from build123d import *

# Parameters (mm, degrees)
SKETCH_1_R                      = 7.5
SKETCH_1_R_2                    = 2.5
EXTRUDE_1_DEPTH                 = 20
SKETCH_2_R                      = 40.75
SKETCH_2_R_2                    = 2.5
EXTRUDE_2_DEPTH                 = 5
EXTRUDE_T_DEPTH                 = 10
EXTRUDE_T_DEPTH_BACK            = 15
SKETCH_3_R                      = 40.75
SKETCH_3_R_2                    = 36.75
SKETCH_4_W                      = 20
SKETCH_4_H                      = 17.5
EXTRUDE_4_DEPTH                 = 70
SKETCH_6_W                      = 8
SKETCH_6_H                      = 17.5
CUT_EXTRUDE_5_DEPTH             = 40
CUT_EXTRUDE_6_REACH             = 101.303
SKETCH_7_R                      = 2.5
CUT_EXTRUDE_7_REACH             = 96.584
SKETCH_8_W                      = 71.008802272
SKETCH_8_H                      = 20.75
CUT_EXTRUDE_7_DIRECTION_2_REACH = 96.584
CUT_EXTRUDE_START               = -55
SKETCH_9_W                      = 20
SKETCH_9_H                      = 5
CUT_EXTRUDE_8_DEPTH             = 55


with BuildPart() as part:
    # Эскиз1 → Вытянуть1 (new body)
    with BuildSketch(Plane(origin=(0, 0, 0), x_dir=(1, 0, 0), z_dir=(0, 1, 0))):
        with Locations(Location((0, 0, 0), (0, 0, 270))):
            Circle(SKETCH_1_R)
        with Locations(Location((0, 0, 0), (0, 0, 270))):
            Circle(SKETCH_1_R_2, mode=Mode.SUBTRACT)
    extrude(amount=EXTRUDE_1_DEPTH)

    # Эскиз2 → Вытянуть2 (add)
    with BuildSketch(Plane(origin=(0, 0, 0), x_dir=(1, 0, 0), z_dir=(0, 1, 0))):
        with Locations(Location((0, 0, 0), (0, 0, 270))):
            Circle(SKETCH_2_R)
        with Locations(Location((0, 0, 0), (0, 0, 270))):
            Circle(SKETCH_2_R_2, mode=Mode.SUBTRACT)
    extrude(amount=EXTRUDE_2_DEPTH)

    # Эскиз3 → t (add, two sides: drawn at the far end of the back side and taken through both)
    with BuildSketch(Plane(origin=(0, 5, 0), x_dir=(1, 0, 0), z_dir=(0, 1, 0)).offset(-EXTRUDE_T_DEPTH_BACK)):
        with Locations(Location((0, 0, 0), (0, 0, 270))):
            Circle(SKETCH_3_R)
        with Locations(Location((0, 0, 0), (0, 0, 270))):
            Circle(SKETCH_3_R_2, mode=Mode.SUBTRACT)
    extrude(amount=EXTRUDE_T_DEPTH + EXTRUDE_T_DEPTH_BACK)

    # Эскиз4 → Вытянуть4 (add)
    with BuildSketch(Plane(origin=(0, 5, 0), x_dir=(1, 0, 0), z_dir=(0, 1, 0))):
        with Locations((0, 11.25)):
            Rectangle(SKETCH_4_W, SKETCH_4_H)
    extrude(amount=EXTRUDE_4_DEPTH)

    # Эскиз6 → Вытянуть5 (cut)
    with BuildSketch(Plane(origin=(0, 75, 0), x_dir=(1, 0, 0), z_dir=(0, 1, 0))):
        with Locations((0, 11.25)):
            Rectangle(SKETCH_6_W, SKETCH_6_H)
    extrude(amount=-CUT_EXTRUDE_5_DEPTH, mode=Mode.SUBTRACT)

    # Вытянуть6: up to this face of the body (flat: up to its plane)
    cut_extrude_6_end = Plane(part.part.faces().sort_by_distance((-10, 40, -11.25))[0])
    # Эскиз7 → Вытянуть6 (cut, up to the picked face)
    with BuildSketch(Plane(origin=(10, 0, 0), x_dir=(0, 0, -1), z_dir=(1, 0, 0)), mode=Mode.PRIVATE) as cut_extrude_6_sk1:
        with Locations((13.75, 45)):
            Circle(SKETCH_7_R)
    cut_extrude_6_tool1 = split(extrude(cut_extrude_6_sk1.sketch, amount=-CUT_EXTRUDE_6_REACH, mode=Mode.PRIVATE), bisect_by=cut_extrude_6_end, keep=Keep.BOTH, mode=Mode.PRIVATE)
    add(cut_extrude_6_tool1.solids().sort_by(Axis((10, 45, -13.75), (-1, 0, 0)))[0], mode=Mode.SUBTRACT)

    # Эскиз8 → Вытянуть7 (cut, up to next)
    with BuildSketch(Plane(origin=(0, 0, 0), x_dir=(1, 0, 0), z_dir=(0, 1, 0)), mode=Mode.PRIVATE) as cut_extrude_7_sk1:
        with Locations((0, 30.375)):
            Rectangle(SKETCH_8_W, SKETCH_8_H)
    cut_extrude_7_tool1 = extrude(cut_extrude_7_sk1.sketch, amount=CUT_EXTRUDE_7_REACH, mode=Mode.PRIVATE) & part.part
    add(cut_extrude_7_tool1.solids().sort_by_distance((0, 0, -30.375))[0], mode=Mode.SUBTRACT)

    # Эскиз8 → Вытянуть7 direction 2 (cut, up to next)
    with BuildSketch(Plane(origin=(0, 0, 0), x_dir=(1, 0, 0), z_dir=(0, 1, 0)), mode=Mode.PRIVATE) as cut_extrude_7_direction_2_sk1:
        with Locations((0, 30.375)):
            Rectangle(SKETCH_8_W, SKETCH_8_H)
    cut_extrude_7_direction_2_tool1 = extrude(cut_extrude_7_direction_2_sk1.sketch, amount=-CUT_EXTRUDE_7_DIRECTION_2_REACH, mode=Mode.PRIVATE) & part.part
    add(cut_extrude_7_direction_2_tool1.solids().sort_by_distance((0, 0, -30.375))[0], mode=Mode.SUBTRACT)

    # Эскиз9 → Вытянуть8 (cut)
    with BuildSketch(Plane(origin=(0, 75, 0), x_dir=(1, 0, 0), z_dir=(0, 1, 0)).offset(CUT_EXTRUDE_START)):
        with Locations((0, 5)):
            Rectangle(SKETCH_9_W, SKETCH_9_H)
    extrude(amount=CUT_EXTRUDE_8_DEPTH, mode=Mode.SUBTRACT)


solid = part.part
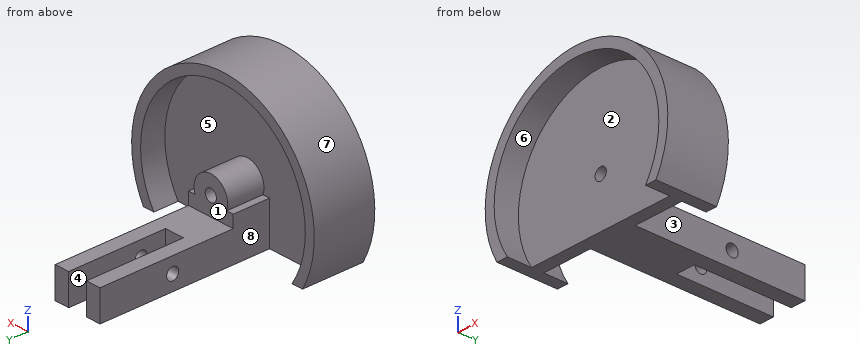
Model file for the job. Use its own axes, mm. Face numbers are marked on the shaded views. A direction names the side the tool comes from. Give positions to 0.01 mm unless a question says otherwise; leave off trailing zeros. Order: outer loops, then holes, each group sorted by start corner. A loop starts at its lowest first (then second) coordinate and runs counter-clockwise, first axis right, second up. Notation, with made-up numbers: (57.25, 88.5) - (114.25, 88.5) arc R29 cw to (114.25, 124.5) - close; hole circle Ø5 at (45.5, 77). An arc over 180 degrees is marked (long way). Return JSON: item names as keys, results as strings.
1) Cut at D-D, the plane z = -13.75. Give the cut face in (x, y), plus the area to 3 significant figures.
Geometry says:
{"outline": "(-38.36, -10) - (-34.08, -10) - (-34.08, 0) - (34.08, 0) - (34.08, -10) - (38.36, -10) - (38.36, 15) - (34.08, 15) - (34.08, 5) - (10, 5) - (10, 42.5) - (4, 42.5) - (4, 35) - (-4, 35) - (-4, 42.5) - (-10, 42.5) - (-10, 5) - (-34.08, 5) - (-34.08, 15) - (-38.36, 15) - close; (-10, 47.5) - (-4, 47.5) - (-4, 75) - (-10, 75) - close; (4, 47.5) - (10, 47.5) - (10, 75) - (4, 75) - close", "area": "1,570 mm²"}
2) Flat gauge pins, fed straight in: P1, Ø22, axis at x = 1, y = 43.5, coming from the +Z side; P2, Ø5, axis at y = 44.5, z = -11.5, coming from the +X side; P3, Ø4, axis at x = 0.5, z = -13, coming from the +Y side. Where does each tip first touch, or does it go through?
Geometry says:
{"P1": "z = -7.5", "P2": "x = 10", "P3": "y = 35"}
3) 3-axis set-ups, long thin cutter, end or side, ignore diameter. For the marked faces 1, 2, 3, 4 and 5: which of +Z, -Z, +X, -X, +Y, -Y reach the whole face in a straight line?
Geometry says:
{"face 1": "+Z, +X, -X, +Y", "face 2": "-Y", "face 3": "-Z, +Y", "face 4": "+Z, -Z, +Y", "face 5": "+Y"}
4) Cut at C-C, the plane y = 53. Give the cut face in (x, z).
Geometry says:
{"outline": "(-10, -20) - (-4, -20) - (-4, -7.5) - (-10, -7.5) - close; (4, -20) - (10, -20) - (10, -7.5) - (4, -7.5) - close"}
5) Cut at B-B, the plane z = 0. Give the cut face in (x, y).
Geometry says:
{"outline": "(-40.75, -10) - (-36.75, -10) - (-36.75, 0) - (-2.5, 0) - (-2.5, 20) - (-7.5, 20) - (-7.5, 5) - (-36.75, 5) - (-36.75, 15) - (-40.75, 15) - close; (2.5, 0) - (36.75, 0) - (36.75, -10) - (40.75, -10) - (40.75, 15) - (36.75, 15) - (36.75, 5) - (7.5, 5) - (7.5, 20) - (2.5, 20) - close"}
6) Pull direction Z, two halves, no side cores. Call the marked faces 6, 7 and 8: pulls with the +Z half, pulls with the -Z half, needs draft (parallel to the pull), parting line crosses it, or undercut.
Geometry says:
{"face 6": "undercut", "face 7": "parting line crosses it", "face 8": "needs draft"}
7) Probe line 1 (X direction, y = 7, z = 0); line 2 (X direction, y = 48, z = -13.5); line 3 (X direction, y = -6, z = 0). List the from-to ranges inside material, lowest first. Write a range as from..to.
Geometry says:
{"line 1": "-40.75..-36.75, -7.5..-2.5, 2.5..7.5, 36.75..40.75", "line 2": "-10..-4, 4..10", "line 3": "-40.75..-36.75, 36.75..40.75"}
8) Cut at A-A, the plane x = 0. Give the cut face in (y, z).
Geometry says:
{"outline": "(-10, 36.75) - (0, 36.75) - (0, 2.5) - (20, 2.5) - (20, 7.5) - (5, 7.5) - (5, 36.75) - (15, 36.75) - (15, 40.75) - (-10, 40.75) - close; (0, -20) - (35, -20) - (35, -7.5) - (20, -7.5) - (20, -2.5) - (0, -2.5) - close"}
